Here's how the part is built. I have some questions about the finished solid (model axes, mm). A direction names the side the tool comes from. Round coordinates to 2 decimals unless told otherwise and drop trailing zeros. Order: outer loops, then holes, each group sorted by start corner. A loop starts at its lowest first (then second) coordinate and runs counter-clockwise, first axis right, second up.
```python
from build123d import *

# Parameters (mm, degrees)
SKETCH1_R               = 11.5
SKETCH1_R_2             = 1.75
BOSS_EXTRUDE1_DEPTH     = 2
CUT_EXTRUDE1_DEPTH      = 17.385969608
CUT_EXTRUDE1_DEPTH_BACK = 17.385969608
SKETCH2_R               = 0.5


with BuildPart() as part:
    # Sketch1 → Boss-Extrude1 (new body)
    with BuildSketch(Plane(origin=(0, 0, 0), x_dir=(1, 0, 0), z_dir=(0, 1, 0))):
        with Locations(Location((0, 0, 0), (0, 0, 270))):
            Circle(SKETCH1_R)
        with Locations(Location((0, 8, 0), (0, 0, 270))):
            Circle(SKETCH1_R_2, mode=Mode.SUBTRACT)
        with Locations(Location((8, 0, 0), (0, 0, 270))):
            Circle(SKETCH1_R_2, mode=Mode.SUBTRACT)
        with Locations(Location((0, -8, 0), (0, 0, 270))):
            Circle(SKETCH1_R_2, mode=Mode.SUBTRACT)
        with Locations(Location((-8, 0, 0), (0, 0, 270))):
            Circle(SKETCH1_R_2, mode=Mode.SUBTRACT)
        Polygon((2.078460969, 3.6), (-2.078460969, 3.6), (-4.156921938, 0), (-2.078460969, -3.6), (2.078460969, -3.6), (4.156921938, 0), align=None, mode=Mode.SUBTRACT)
    extrude(amount=BOSS_EXTRUDE1_DEPTH)

    # Sketch2 → Cut-Extrude1 (cut, two sides: drawn at the far end of the back side and taken through both)
    with BuildSketch(Plane.XZ.offset(-CUT_EXTRUDE1_DEPTH_BACK)):
        with Locations((-2.078460969, 3.6)):
            Circle(SKETCH2_R)
        with Locations((2.078460969, 3.6)):
            Circle(SKETCH2_R)
        with Locations((4.156921938, 0)):
            Circle(SKETCH2_R)
        with Locations((2.078460969, -3.6)):
            Circle(SKETCH2_R)
        with Locations((-2.078460969, -3.6)):
            Circle(SKETCH2_R)
        with Locations((-4.156921938, 0)):
            Circle(SKETCH2_R)
    extrude(amount=CUT_EXTRUDE1_DEPTH + CUT_EXTRUDE1_DEPTH_BACK, mode=Mode.SUBTRACT)


solid = part.part
```
1) I'm going to push flat-ended pins straight in: pin 1 (1 mm diameter, centred on x = 2, y = 1, fed in from +Z); pin 2 (3 mm diameter, centred on x = 0, z = -8, fed in from -Y). Where does each tip first touch, or does it pass through?
2) If we section it at A-A (y = 0.85): Write out the boundary of the cut face in (x, z), plus the area to 3 significant figures.
3) I need wall thicknesses on line 1 (Z direction, x = -0.75, y = 1.95); line 2 (Z direction, x = -1.25, y = 0.85); line 3 (X direction, y = 0.3, z = 1). Which ranges of each line are inside material? Lowest first, please.
4) For faces 1 (the flat face through (0, 1, -3.6)), 2 (the flat face through (3, 2, -3)), which set-ups out of +Z, -Z, +X, -X, +Y, -Y let a thin tool reach every point of the face, with its end or its side?
5) We'd pull the mould along X, two halves only. Please class faces 3 (the cylindrical face through (-2.341, 1.014, -4.025)), 4 (the flat face through (3, 0, -3)), 5 (the cylindrical face through (9.7, 0.99, 6.18)): +X half, -X half, draft (parallel to the pull), parting line (faces both ways), or undercut.
6) If we section it at C-C (z = -7.5): Write out the boundary of the cut face in (x, y).
7) If we section it at B-B (x = 0): Write out the boundary of the cut face in (y, z), plus the area to 3 significant figures.
8) If we section it at D-D (x = 8): Write out the boundary of the cut face in (y, z), plus the area to 3 significant figures.
Solutions:
1. pin 1: stops at z = 11.4
1. pin 2: passes through
2. outline: circle Ø23 at (0, 0); hole circle Ø3.5 at (-8, 0); hole (-3.91, -0.43) - (-2.33, -3.17) arc R0.5 ccw (long way) to (-1.58, -3.6) - (1.58, -3.6) arc R0.5 ccw (long way) to (2.33, -3.17) - (3.91, -0.43) arc R0.5 ccw (long way) to (3.91, 0.43) - (2.33, 3.17) arc R0.5 ccw (long way) to (1.58, 3.6) - (-1.58, 3.6) arc R0.5 ccw (long way) to (-2.33, 3.17) - (-3.91, 0.43) arc R0.5 ccw (long way) to start; hole circle Ø3.5 at (0, -8); hole circle Ø3.5 at (0, 8); hole circle Ø3.5 at (8, 0)
2. area: 329 mm2
3. line 1: z = -11.48 to -9.58, -6.42 to -3.6, 3.6 to 6.42, 9.58 to 11.48
3. line 2: z = -11.43 to -9.22, -6.78 to -3.6, 3.6 to 6.78, 9.22 to 11.43
3. line 3: x = -11.46 to -9.44, -6.56 to -3.58, 3.58 to 6.56, 9.44 to 11.46
4. face 1: +Y, -Y
4. face 2: +Z, -Z, +X, -X, +Y
5. face 3: undercut
5. face 4: draft
5. face 5: parting line
6. outline: (-8.72, 0) - (-1.68, 0) - (-1.68, 2) - (-8.72, 2) - close; (1.68, 0) - (8.72, 0) - (8.72, 2) - (1.68, 2) - close
7. outline: (0, -11.5) - (2, -11.5) - (2, -9.75) - (0, -9.75) - close; (0, -6.25) - (2, -6.25) - (2, -3.6) - (0, -3.6) - close; (0, 3.6) - (2, 3.6) - (2, 6.25) - (0, 6.25) - close; (0, 9.75) - (2, 9.75) - (2, 11.5) - (0, 11.5) - close
7. area: 17.6 mm2
8. outline: (0, -8.26) - (2, -8.26) - (2, -1.75) - (0, -1.75) - close; (0, 1.75) - (2, 1.75) - (2, 8.26) - (0, 8.26) - close
8. area: 26.0 mm2
